Here's the drawing with two shaded views (mm, measured from the low corner). I have some questions. A direction names the side the tool comes from. Give positions to 0.01 mm unless a question says otherwise; leave off trailing zeros. Order: outer loops, then holes, each group sorted by start corner. A loop starts at its lowest first (then second) coordinate and runs counter-clockwise, first axis right, second up. Notation, with made-up numbers: M 66.5,62.5 L 118.5,62.5 A13 ccw 118.5,75.5 Z; hole C 4,11 d6. An arc over 180 degrees is marked long. Use a Markdown table: item, result. Add a question column.
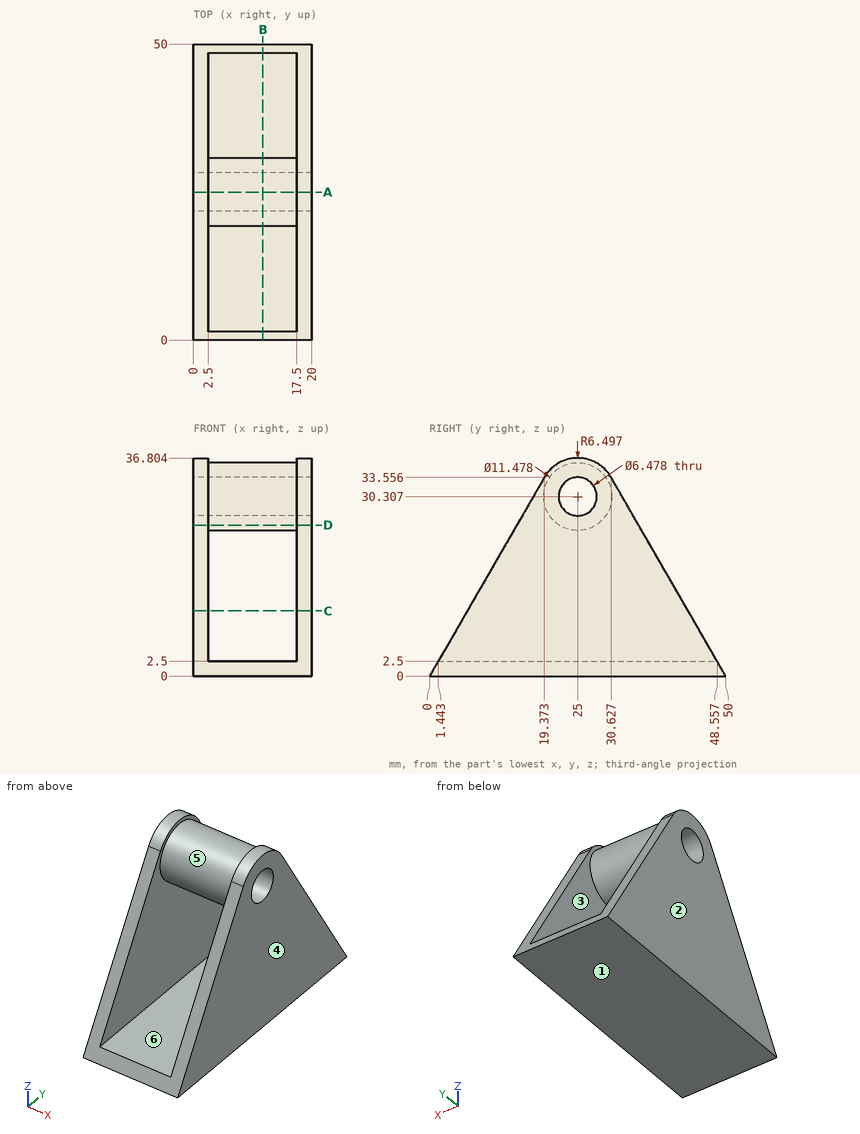
1. I need wall thicknesses on L1, parallel to Z at x = 6.5, y = 25; L2, parallel to X at y = 14.5, z = 17; L3, parallel to Z at x = 5, y = 46. Which ranges of each line are inside material? Lowest first, please. Write a range as [from, to].
2. If we section it at B-B, the plane x = 11.75: List the corners of the cut face in (y, z) for me.
3. If we section it at D-D, the plane z = 25.5: List the corners of the cut face in (x, y) for me (1 decimal).
4. We'd pull the mould along Z, two halves only. Please class the marked faces 1, 2 and 3: +Z half, -Z half, draft (parallel to the pull), parting line (faces both ways), or undercut.
5. If we section it at C-C, the plane z = 11: List the corners of the cut face in (x, y) for me.
6. If we section it at A-A, the plane y = 25: List the corners of the cut face in (x, z) for me (1 decimal), then the cut area to 3 significant figures.
7. On a 3-axis mill with a long thin cutter (end or side, diameter ignored), from which of +Z, -Z, +X, -X, +Y, -Y can I reach the whole of each face in a straight line? I mean the marked faces 4, 5 and 6. Say none if no direction works.
8. Will these pins go through, and if not, where does the flat tip stop? pin 1 (10 mm diameter, centred on x = 2.5, y = 30.5, fed in from +Z) (1 decimal); pin 2 (6 mm diameter, centred on x = 15.5, z = 21, fed in from +Y); pin 3 (3 mm diameter, centred on x = 17.5, z = 23.5, fed in from +Y).
Geometry results:
| question | item | result |
|---|---|---|
| 1 | L1 | z = [0, 2.5], [24.57, 27.07], [33.55, 36.05] |
| 1 | L2 | x = [0, 2.5], [17.5, 20] |
| 1 | L3 | z = [0, 2.5] |
| 2 | outline | M 0,0 L 50,0 L 48.56,2.5 L 1.44,2.5 Z; C 25,30.31 d11.48; hole C 25,30.31 d6.48 |
| 3 | outline | M 0,14.7 L 2.5,14.7 L 2.5,21.9 L 17.5,21.9 L 17.5,14.7 L 20,14.7 L 20,35.3 L 17.5,35.3 L 17.5,28.1 L 2.5,28.1 L 2.5,35.3 L 0,35.3 Z |
| 4 | face 1 | -Z half |
| 4 | face 2 | draft |
| 4 | face 3 | undercut |
| 5 | outline | M 0,6.35 L 2.5,6.35 L 2.5,43.65 L 0,43.65 Z; M 17.5,6.35 L 20,6.35 L 20,43.65 L 17.5,43.65 Z |
| 6 | outline | M 0,0 L 20,0 L 20,27.1 L 0,27.1 Z; M 0,33.5 L 20,33.5 L 20,36.8 L 17.5,36.8 L 17.5,36 L 2.5,36 L 2.5,36.8 L 0,36.8 Z; hole M 2.5,2.5 L 17.5,2.5 L 17.5,24.6 L 2.5,24.6 Z |
| 6 | area | 264 mm^2 |
| 7 | face 4 | +Z, -Z, +X, +Y, -Y |
| 7 | face 5 | none |
| 7 | face 6 | +Y, -Y |
| 8 | pin 1 | stops at z = 36.8 |
| 8 | pin 2 | stops at y = 39.17 |
| 8 | pin 3 | stops at y = 37.3 |
